from build123d import *

# Parameters (mm, degrees)
SKETCH1_R           = 3
BOSS_EXTRUDE1_DEPTH = 3


with BuildPart() as part:
    # Sketch1 → Boss-Extrude1 (new body)
    with BuildSketch(Plane.XY):
        with BuildLine():
            Line((162.640616578, -47.437292702), (141.367093537, -59.798809878))
            ThreePointArc((141.367093537, -59.798809878), (136.844335561, -74.68318626), (151.728711943, -79.205944236))
            Line((151.728711943, -79.205944236), (152.402593626, -78.814873748))
            Line((152.402593626, -78.814873748), (173.688379763, -66.462196747))
            Line((173.688379763, -66.462196747), (216.929531333, -41.352308153))
            ThreePointArc((216.929531333, -41.352308153), (220.918167116, -26.315991874), (205.881850837, -22.32735609))
            Line((205.881850837, -22.32735609), (162.640616578, -47.437292702))
        make_face()
        with Locations((146.547901788, -69.502375418)):
            Circle(SKETCH1_R, mode=Mode.SUBTRACT)
        with Locations((168.167159933, -56.948185788)):
            Circle(SKETCH1_R, mode=Mode.SUBTRACT)
        with Locations((211.405691085, -31.839832122)):
            Circle(SKETCH1_R, mode=Mode.SUBTRACT)
    extrude(amount=BOSS_EXTRUDE1_DEPTH)


solid = part.part
Verification items for the finished model (mm, model axes). Coordinates: 2 decimals unless noted, no trailing zeros. Order: outer loops, then holes, each group sorted by start corner. A loop starts at its lowest first (then second) coordinate and runs counter-clockwise, first axis right, second up.
1. Sectioned sample at B-B, the plane z = 2.55. Record the cut outline in (x, y), and give its area (3 significant figures).
Results found:
outline: (141.37, -59.8) arc R11 ccw to (151.73, -79.21) - (173.69, -66.46) - (216.93, -41.35) arc R11 ccw to (205.88, -22.33) - (162.64, -47.44) - close; hole circle Ø6 at (146.55, -69.5); hole circle Ø6 at (168.17, -56.95); hole circle Ø6 at (211.41, -31.84)
area: 1,950 mm2
2. Sectioned sample at C-C, the plane y = -56. Record the cut outline in (x, z).
Results found:
outline: (147.9, 0) - (165.32, 0) - (165.32, 3) - (147.9, 3) - close; (171.01, 0) - (191.71, 0) - (191.71, 3) - (171.01, 3) - close
3. Scan lines: line 1 (X direction, y = -71.5, z = 1.85); line 2 (Y direction, x = 166.5, z = 2.85); line 3 (Y direction, x = 212, z = 0.5). Record each from-to range of solid material in increasing order.
Results found:
line 1: x = 135.73 to 144.31, 148.79 to 165.01
line 2: y = -70.63 to -59.44, -54.45 to -45.2
line 3: y = -44.21 to -34.78, -28.9 to -20.86
4. Sectioned sample at A-A, the plane y = -33.5. Record the cut outline in (x, z).
Results found:
outline: (186.64, 0) - (208.91, 0) - (208.91, 3) - (186.64, 3) - close; (213.9, 0) - (222.28, 0) - (222.28, 3) - (213.9, 3) - close
5. Sectioned sample at D-D, the plane x = 157. Record the cut outline in (y, z), and give its area (3 significant figures).
Results found:
outline: (-76.15, 0) - (-50.71, 0) - (-50.71, 3) - (-76.15, 3) - close
area: 76.3 mm2
6. Release check for a two-part mould opening along Y. For faces 1 (the face through (136.733, -74.469, 1.479)), 2 (the face through (178, -50, 3)), 3 (the face through (208.41, -31.71, 1.48)) record: +Y half, -Y half, draft (parallel to the pull), parting line (faces both ways), or undercut.
Results found:
face 1: parting line
face 2: draft
face 3: undercut
7. Go/stop test with a flat-tipped pin: pin 1 Ø8 at (x, y) = (211.41, -31.84) entering from +Z. Record where the tip stops, or that it passes through.
Results found:
pin 1: stops at z = 3
